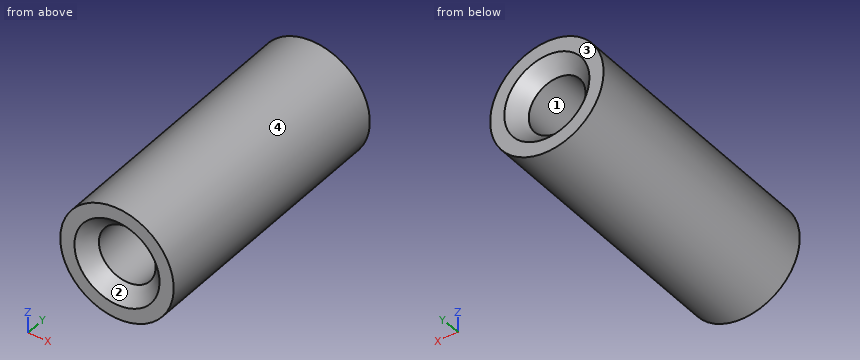
Autodesk Inventor part; units mm, degrees
ref_plane "YZ Plane" through (0, 0, 0) normal (1, 0, 0) x (0, 1, 0)
ref_plane "XZ Plane" through (0, 0, 0) normal (0, 1, 0) x (-1, 0, 0)
ref_plane "XY Plane" through (0, 0, 0) normal (0, 0, 1) x (1, 0, 0)
sketch "スケッチ1" plane through (0, 0, 0) normal (0, 1, 0) x (-1, 0, 0)
  circle A0 centre (0, 0) radius 2
  dimension "d0" = 4
extrude "押し出し1" add sketch "スケッチ1" along normal blind 9.56
sketch "スケッチ2" plane through (0, 9.56, 0) normal (0, 1, 0) x (1, 0, 0)
  point P0 (0, 0)
hole "穴1" at (0, 9.56, 0) direction (0, -1, 0) diameter 2 end through all countersink diameter 3 countersink angle 90
sketch "スケッチ3" plane through (0, 0, 0) normal (0, -1, 0) x (1, 0, 0)
  point P0 (0, 0)
hole "穴2" at (0, 0, 0) direction (0, 1, 0) diameter 2 end through all countersink diameter 3 countersink angle 90
properties part number "shaft" material "鉄、鋳鉄"
Work out the finished part from the listing and answer in its coordinate system (mm). Face numbers are marked on the shaded views. Give positions to 0.01 mm unless a question says otherwise; leave off trailing zeros. Order: outer loops, then holes, each group sorted by start corner. A loop starts at its lowest first (then second) coordinate and runs counter-clockwise, first axis right, second up. Notation, with made-up numbers: (-11, 44) -> (30, 44) arc R19 ccw to (30, 56) -> close; hole circle Ø3 at (39, -14.5). An arc over 180 degrees is marked (long way). Answer as a JSON object with one key per item and string values. Group by question number.
1. Consider line 1 along Z through (x, y) = (0, 3); line 2 along Z through (x, y) = (0.55, 8); line 3 along X through (y, z) = (1.5, -0.4). Determine where each line is inside the solid, lowest interval first. Write a range as [from, to].
2. The mould has two halves that part along X. Classify the marked faces 1, 2, 3 and 4: released by +X, released by -X, zero draft, split by the parting line, or undercut.
3. Flat-ended cylindrical pins translate along their axes: pin 1 Ø1 at (y, z) = (4.5, -1) entering from +X; pin 2 Ø1.8 at (x, z) = (0, 0) entering from -Y; pin 3 Ø1.5 at (x, y) = (-1, 5) entering from -Z; pin 4 Ø2 at (y, z) = (5.5, 1.5) entering from -X. Find the tip coordinate at first contact, or state that the pin passes through.
4. Section C-C on y = 3.25 is taken. Determine the outline of the cut face in (x, z).
5. Section B-B on x = 0 is taken. Determine the outline of the cut face in (y, z), plus the area to 3 significant figures.
6. Section A-A on z = 0 is taken. Determine the outline of the cut face in (x, y), plus the area to 3 significant figures.
Result sheet:
{
 "1": {"line 1": "z = [-2, -1], [1, 2]", "line 2": "z = [-1.92, -0.84], [0.84, 1.92]", "line 3": "x = [-1.96, -0.92], [0.92, 1.96]"},
 "2": {"face 1": "undercut", "face 2": "undercut", "face 3": "zero draft", "face 4": "split by the parting line"},
 "3": {"pin 1": "stops at x = 1.94", "pin 2": "passes through", "pin 3": "stops at z = -1.98", "pin 4": "stops at x = -1.94"},
 "4": {"outline": "circle Ø4 at (0, 0); hole circle Ø2 at (0, 0)"},
 "5": {"outline": "(0, -2) -> (9.56, -2) -> (9.56, -1.5) -> (9.06, -1) -> (0.5, -1) -> (0, -1.5) -> close; (0, 1.5) -> (0.5, 1) -> (9.06, 1) -> (9.56, 1.5) -> (9.56, 2) -> (0, 2) -> close", "area": "18.6 mm^2"},
 "6": {"outline": "(-2, 0) -> (-1.5, 0) -> (-1, 0.5) -> (-1, 9.06) -> (-1.5, 9.56) -> (-2, 9.56) -> close; (1, 0.5) -> (1.5, 0) -> (2, 0) -> (2, 9.56) -> (1.5, 9.56) -> (1, 9.06) -> close", "area": "18.6 mm^2"}
}
